Check sheet for the modelled part. Datum: model origin and axes. Units: mm. A direction names the side the tool comes from. Give positions to 0.01 mm unless a question says otherwise; leave off trailing zeros. Loops run counter-clockwise (first coordinate to the right, second up) from the corner with the lowest first, then second, coordinate; pieces in that order, holes last. Notation, with made-up numbers: (32, 7.25) -> (78, 7.25) arc R12 cw to (78, 30.25) -> close; hole circle Ø4 at (76.5, 4). An arc over 180 degrees is marked (long way). Write each question's results on one line, items separated by ' | '. Start each with the question number.
1. Cross-section at B-B on x = 62. Record the boundary of the cut face in (y, z), and give its area (3 significant figures).
2. Material ranges on L1, parallel to Z at x = 61.5, y = -18.5, recorded low to high. Write a range as from..to.
3. Cross-section at A-A on y = -10.5. Record the boundary of the cut face in (x, z).
4. Gauge pin test, flat ends, axial feed: pin 1 Ø3 at (y, z) = (22, 96) entering from +X; pin 2 Ø1.4 at (y, z) = (21.5, 97) entering from -X; pin 3 Ø1.1 at (y, z) = (20.5, 98.5) entering from +X; pin 4 Ø2.5 at (x, y) = (-58.5, -21.5) entering from -Z. Record the tip position at first contact, or that the pin passes through.
5. Mould release check, pull along Z, two halves, no side actions. Record for faces 1 (the face through (-58.9, 24.05, 98.2)), 2 (the face through (-58, -22, 98)), 3 (the face through (-58, -22, 99)): +Z half, -Z half, draft (parallel to the pull), parting line (faces both ways), or undercut.
6. Tool access check on faces 4 (the face through (-58.9, -24.05, 98.2)), 5 (the face through (-58.9, 19.45, 98.2)), 6 (the face through (-61, -22, 96)), 7 (the face through (-1, -31.9, 46)), 8 (the face through (-62, 22, 97)). Record the directions out of +Z, -Z, +X, -X, +Y, -Y that give a thin tool (end or side, any length) a straight path to the whole face; none if there is none.
from build123d import *

# Parameters (mm, degrees)
F0_W     = 150
F0_H     = 63.8
F1_DEPTH = 94
F4_DEPTH = 2.3
F5_R     = 1


# Not quite as in the source:
# - a pattern or mirror of a feature is missing from the dataset's text; its kind, count and spacing are read off the source's solid


with BuildPart() as f1:
    # F0 (on Top) → F1 (new body)
    with BuildSketch(Plane.XY):
        Rectangle(F0_W, F0_H)
    extrude(amount=F1_DEPTH)

    # F3 (on offset) → F4 (join, symmetric)
    with BuildSketch(Plane.XZ.offset(21.75)):
        Polygon((-62, 99), (-62, 94), (-61, 94), (-61, 98), (-54, 98), (-54, 99), align=None)
    f4 = extrude(amount=F4_DEPTH, both=True)

    # F4_copies: F4 across plane
    add(f4.mirror(Plane.ZX))

    # F5
    f5_edges = [f1.edges().sort_by_distance(p)[0] for p in [
        (0, -31.9, 94),
        (75, 0, 94),
        (0, 31.9, 94),
        (-75, 0, 94),
        (-75, -31.9, 47),
        (75, -31.9, 47),
        (0, -31.9, 0),
        (75, 31.9, 47),
        (75, 0, 0),
        (-75, 31.9, 47),
        (0, 31.9, 0),
        (-75, 0, 0),
    ]]
    fillet(f5_edges, radius=F5_R)


solid = f1.part
Geometry says:
1) outline: (-31.9, 1) arc R1 ccw to (-30.9, 0) -> (30.9, 0) arc R1 ccw to (31.9, 1) -> (31.9, 93) arc R1 ccw to (30.9, 94) -> (-30.9, 94) arc R1 ccw to (-31.9, 93) -> close | area: 6,000 mm^2
2) L1: 0..94
3) outline: (-75, 1) arc R1 ccw to (-74, 0) -> (74, 0) arc R1 ccw to (75, 1) -> (75, 93) arc R1 ccw to (74, 94) -> (-74, 94) arc R1 ccw to (-75, 93) -> close
4) pin 1: x = -61 | pin 2: x = -62 | pin 3: x = -54 | pin 4: z = 0
5) face 1: draft | face 2: undercut | face 3: +Z half
6) face 4: +Z, +X, -X, -Y | face 5: +Z, +X, -X | face 6: +X, +Y, -Y | face 7: +Z, -Z, +X, -X, -Y | face 8: +Z, -X, +Y, -Y
